```python
from build123d import *

# Parameters (mm, degrees)
F0_W     = 152.4
F0_H     = 25.4
F0_H_2   = 50.8
F1_DEPTH = 10
F2_W     = 106.68
F2_H     = 50.8
F3_DEPTH = 25.4


with BuildPart() as f1:
    # F0 (on Top) → F1 (new body)
    with BuildSketch(Plane.XY):
        Polygon((88.9, -76.2), (88.9, 25.4), (76.2, 25.4), (76.2, 0), (-76.2, 0), (-76.2, 25.4), (-88.9, 25.4), (-88.9, -76.2), align=None)
        with Locations((0, 12.7)):
            Rectangle(F0_W, F0_H)
        with Locations((0, 50.8)):
            Rectangle(F0_W, F0_H_2)
    extrude(amount=F1_DEPTH)

    # F2 (on face) → F3 (cut)
    with BuildSketch(Plane.XY.offset(10)):
        with Locations((0, -50.8)):
            Rectangle(F2_W, F2_H)
    extrude(amount=-F3_DEPTH, mode=Mode.SUBTRACT)


solid = f1.part
```
Source: CAD feature listing. Evaluate the final solid. Frame: model axes, mm. A direction names the side the tool comes from. Round coordinates to 2 decimals unless told otherwise and drop trailing zeros. Loops run counter-clockwise (first coordinate to the right, second up) from the corner with the lowest first, then second, coordinate; pieces in that order, holes last. Notation, with made-up numbers: M 87,47 L 145,47 A21 ccw 145,56 Z; hole C 45,-17.75 d8. An arc over 180 degrees is marked long. Use a Markdown table: item, result. Add a question column.
1. Cut plane A-A, the plane y = -37.5. Output: boundary loops of the cut face in (x, z), and give its area (3 significant figures).
2. Ray query, line 1 along X through (y, z) = (-31, 7.75); line 2 along X through (y, z) = (42, 2); line 3 along Y through (x, z) = (49, 5.25). Return the intervals inside material, ascending. Write a range as [from, to].
3. Set-up query: faces 1 (the flat face through (83, 25.4, 5)), 2 (the flat face through (-82, 25.4, 5)), 3 (the flat face through (53.34, -51, 5)), 4 (the flat face through (-1, 1, 10)). Return all of +Z, -Z, +X, -X, +Y, -Y with unobstructed straight access to the full face (end or side cutting, diameter ignored); none if empty.
4. Pull-direction query (X, two-part tool) for faces 5 (the flat face through (76.2, 50, 5)), 6 (the flat face through (-1, -25.4, 5)), 7 (the flat face through (-76.2, 50, 5)); classes: +X half, -X half, draft (parallel to the pull), parting line (faces both ways), or undercut.
5. Cut plane D-D, the plane y = 44. Output: boundary loops of the cut face in (x, z).
6. Cut plane C-C, the plane x = -26. Output: boundary loops of the cut face in (y, z).
7. Cut plane B-B, the plane z = 1.5. Output: boundary loops of the cut face in (x, y).
8. Contact query for flat-ended pins moving along their axis: pin 1 (6 mm diameter, centred on y = 59, z = 8.5, fed in from +X); pin 2 (3 mm diameter, centred on x = 4, z = 3, fed in from -Y); pin 3 (3 mm diameter, centred on y = 49, z = 4.5, fed in from -X). Output: stop coordinate, or through.
Solution:
| question | item | result |
|---|---|---|
| 1 | outline | M -88.9,0 L -53.34,0 L -53.34,10 L -88.9,10 Z; M 53.34,0 L 88.9,0 L 88.9,10 L 53.34,10 Z |
| 1 | area | 711 mm2 |
| 2 | line 1 | x = [-88.9, -53.34], [53.34, 88.9] |
| 2 | line 2 | x = [-76.2, 76.2] |
| 2 | line 3 | y = [-25.4, 76.2] |
| 3 | face 1 | +Z, -Z, +X, +Y |
| 3 | face 2 | +Z, -Z, -X, +Y |
| 3 | face 3 | +Z, -Z, -Y |
| 3 | face 4 | +Z, +X, -X, +Y, -Y |
| 4 | face 5 | +X half |
| 4 | face 6 | undercut |
| 4 | face 7 | -X half |
| 5 | outline | M -76.2,0 L 76.2,0 L 76.2,10 L -76.2,10 Z |
| 6 | outline | M -25.4,0 L 76.2,0 L 76.2,10 L -25.4,10 Z |
| 7 | outline | M -88.9,-76.2 L -53.34,-76.2 L -53.34,-25.4 L 53.34,-25.4 L 53.34,-76.2 L 88.9,-76.2 L 88.9,25.4 L 76.2,25.4 L 76.2,76.2 L -76.2,76.2 L -76.2,25.4 L -88.9,25.4 Z |
| 8 | pin 1 | stops at x = 76.2 |
| 8 | pin 2 | stops at y = -25.4 |
| 8 | pin 3 | stops at x = -76.2 |
